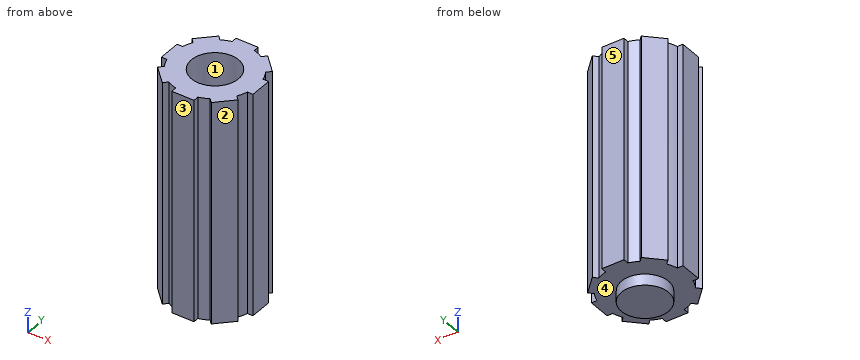
```python
from build123d import *

# Parameters (mm, degrees)
F0_R     = 10.7696
F1_DEPTH = 2.54
F2_DEPTH = 101.6
F3_DEPTH = 5.08


with BuildPart() as f1:
    # F0 (on Top) → F1 (new body)
    with BuildSketch(Plane.XY):
        Circle(F0_R)
    extrude(amount=F1_DEPTH)

    # F0 (on Top) → F2 (join)
    with BuildSketch(Plane.XY):
        with BuildLine():
            Line((5.08, 20.900177), (-5.08, 20.900177))
            Line((-5.08, 20.900177), (-5.08, 18.360177))
            ThreePointArc((-5.08, 18.360177), (-7.290119, 17.599905), (-9.390503, 16.574708))
            Line((-9.390503, 16.574708), (-11.186554, 18.370759))
            Line((-11.186554, 18.370759), (-18.370759, 11.186554))
            Line((-18.370759, 11.186554), (-16.574708, 9.390503))
            ThreePointArc((-16.574708, 9.390503), (-17.599905, 7.290119), (-18.360177, 5.08))
            Line((-18.360177, 5.08), (-20.900177, 5.08))
            Line((-20.900177, 5.08), (-20.900177, -5.08))
            Line((-20.900177, -5.08), (-18.360177, -5.08))
            ThreePointArc((-18.360177, -5.08), (-17.599905, -7.290119), (-16.574708, -9.390503))
            Line((-16.574708, -9.390503), (-18.370759, -11.186554))
            Line((-18.370759, -11.186554), (-11.186554, -18.370759))
            Line((-11.186554, -18.370759), (-9.390503, -16.574708))
            ThreePointArc((-9.390503, -16.574708), (-7.290119, -17.599905), (-5.08, -18.360177))
            Line((-5.08, -18.360177), (-5.08, -20.900177))
            Line((-5.08, -20.900177), (5.08, -20.900177))
            Line((5.08, -20.900177), (5.08, -18.360177))
            ThreePointArc((5.08, -18.360177), (7.290119, -17.599905), (9.390503, -16.574708))
            Line((9.390503, -16.574708), (11.186554, -18.370759))
            Line((11.186554, -18.370759), (18.370759, -11.186554))
            Line((18.370759, -11.186554), (16.574708, -9.390503))
            ThreePointArc((16.574708, -9.390503), (17.599905, -7.290119), (18.360177, -5.08))
            Line((18.360177, -5.08), (20.900177, -5.08))
            Line((20.900177, -5.08), (20.900177, 5.08))
            Line((20.900177, 5.08), (18.360177, 5.08))
            ThreePointArc((18.360177, 5.08), (17.599905, 7.290119), (16.574708, 9.390503))
            Line((16.574708, 9.390503), (18.370759, 11.186554))
            Line((18.370759, 11.186554), (11.186554, 18.370759))
            Line((11.186554, 18.370759), (9.390503, 16.574708))
            ThreePointArc((9.390503, 16.574708), (7.290119, 17.599905), (5.08, 18.360177))
            Line((5.08, 18.360177), (5.08, 20.900177))
        make_face()
        Circle(F0_R, mode=Mode.SUBTRACT)
    extrude(amount=F2_DEPTH)

    # F0 (on Top) → F3 (join)
    with BuildSketch(Plane.XY):
        Circle(F0_R)
    extrude(amount=-F3_DEPTH)


solid = f1.part
```
Could you check a few things on this model? Use its own coordinates, in mm. Face numbers are marked on the shaded views. A direction names the side the tool comes from. Round coordinates to 2 decimals unless told otherwise and drop trailing zeros. Loops run counter-clockwise (first coordinate to the right, second up) from the corner with the lowest first, then second, coordinate; pieces in that order, holes last. Notation, with made-up numbers: (67, -26) - (98, -26) arc R18 cw to (98, -5) - close; hole circle Ø10 at (64.5, 81.5). An arc over 180 degrees is marked (long way). Answer in a Markdown table with one row per item. Add a question column.
(1) I need wall thicknesses on line 1 along Z through (x, y) = (7.5, 8); line 2 along Y through (x, z) = (0, 77); line 3 along Z through (x, y) = (-4.5, 7.5). Which ranges of each line are inside material? Lowest first, please.
(2) If we section it at B-B (x = 0): Please give me the cut outline in (y, z), plus the area to 3 significant figures.
(3) I'm going to push flat-ended pins straight in: pin 1 (3 mm diameter, centred on x = 11, z = 45, fed in from +Y); pin 2 (12 mm diameter, centred on y = -13.5, z = 51, fed in from +X); pin 3 (2 mm diameter, centred on y = -19.5, z = 57.5, fed in from -X). Where does each tip first touch, or does it pass through?
(4) If we section it at D-D (x = -14.5): Please give me the cut outline in (y, z).
(5) For the marked faces 4 and 5, which set-ups out of +Z, -Z, +X, -X, +Y, -Y let a thin tool reach every point of the face, with its end or its side?
(6) If we mould it in two halves opening along X, with no side actions, what happens to the marked faces 1, 2 and 3? For each: pulls with the +X half, pulls with the -X half, needs draft (parallel to the pull), parting line crosses it, or undercut.
Model answer:
| question | item | result |
|---|---|---|
| 1 | line 1 | z = 0 to 101.6 |
| 1 | line 2 | y = -20.9 to -10.77, 10.77 to 20.9 |
| 1 | line 3 | z = -5.08 to 2.54 |
| 2 | outline | (-20.9, 0) - (-10.77, 0) - (-10.77, -5.08) - (10.77, -5.08) - (10.77, 0) - (20.9, 0) - (20.9, 101.6) - (10.77, 101.6) - (10.77, 2.54) - (-10.77, 2.54) - (-10.77, 101.6) - (-20.9, 101.6) - close |
| 2 | area | 2,220 mm² |
| 3 | pin 1 | stops at y = 18.37 |
| 3 | pin 2 | stops at x = 18.37 |
| 3 | pin 3 | stops at x = -5.08 |
| 4 | outline | (-15.06, 0) - (15.06, 0) - (15.06, 101.6) - (-15.06, 101.6) - close |
| 5 | face 4 | -Z |
| 5 | face 5 | +Z, -Z, +X, -X, +Y |
| 6 | face 1 | undercut |
| 6 | face 2 | pulls with the +X half |
| 6 | face 3 | needs draft |
